Autodesk Inventor part; units mm, degrees
ref_plane "YZ Plane" through (0, 0, 0) normal (1, 0, 0) x (0, 1, 0)
ref_plane "XZ Plane" through (0, 0, 0) normal (0, 1, 0) x (-1, 0, 0)
ref_plane "XY Plane" through (0, 0, 0) normal (0, 0, 1) x (1, 0, 0)
sketch "Sketch1" plane through (0, 0, 0) normal (0, 1, 0) x (-1, 0, 0)
  line L0 (0, 0) -> (-358.4448, 0)
  line L1 (0, 0) -> (-358.4448, 0) construction
  line L2 (0, 0) -> (-358.4448, 0) construction
  line L3 (0, 25.4) -> (-358.4448, 25.4)
  line L4 (-358.4448, -25.4) -> (0, -25.4)
  arc A0 (0, -25.4) -> (0, 25.4) centre (0, 0) ccw
  arc A1 (-358.4448, 25.4) -> (-358.4448, -25.4) centre (-358.4448, 0) ccw
  circle A2 centre (0, 0) radius 14.2875
  circle A3 centre (-358.4448, 0) radius 14.2875
  point P0 (-179.2224, 0)
  point P1 (-179.2224, 0)
  dimension "d0" = 358.4448
  dimension "d8" = 50.8
  dimension "d9" = 28.575
  dimension "d10" = 28.575
extrude "Extrusion1" add sketch "Sketch1" along normal blind 6.35
properties part number "4-bar intake (14.112) bar"
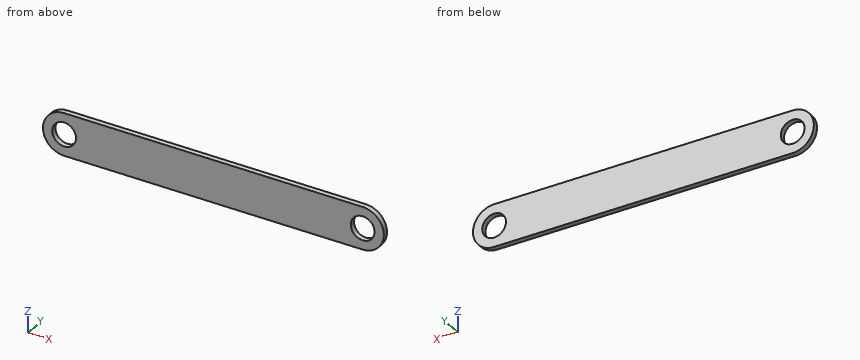
CAD build for the part. Positions are in the model's coordinates, mm. Give positions to 0.01 mm unless a question says otherwise; leave off trailing zeros. Write each loop counter-clockwise with the first axis right and the second up, starting at its lowest first coordinate (ties: lowest second). Pieces come first, ordered by that corner, then holes. Notation, with made-up numbers: M 11.5,46.5 L 64.5,46.5 A32 ccw 64.5,84.5 Z; hole C 18,39 d10. An arc over 180 degrees is marked long. Return JSON: item names as keys, results as strings. Group by question number.
(1) Drill centre lines: L1, parallel to X at y = 1.5, z = 1; L2, parallel to Z at x = 0, y = 2.5; L3, parallel to X at y = 5.75, z = -2. Where is each one in solid material? Low to high. Write a range as [from, to].
(2) Band-saw the part on A-A (z = 0). Give the cut face in (x, y).
(3) Flat gauge pins, fed straight in: pin 1 Ø23 at (x, z) = (0, 0) entering from +Y; pin 2 Ø2 at (y, z) = (2.5, -19) entering from -X; pin 3 Ø1.5 at (y, z) = (1, -19) entering from +X; pin 4 Ø1 at (y, z) = (4, 5.5) entering from +X. Where does each tip first touch, or does it go through?
(4) Band-saw the part on B-B (y = 1.5). Give the cut face in (x, z) (1 decimal), and give its area (3 significant figures).
(5) Band-saw the part on C-C (z = 18.5). Give the cut face in (x, y), and give its area (3 significant figures).
Entries:
{
 "1": {"L1": "x = [-25.38, -14.25], [14.25, 344.19], [372.7, 383.83]", "L2": "z = [-25.4, -14.29], [14.29, 25.4]", "L3": "x = [-25.32, -14.15], [14.15, 344.3], [372.59, 383.77]"},
 "2": {"outline": "M -25.4,0 L -14.29,0 L -14.29,6.35 L -25.4,6.35 Z; M 14.29,0 L 344.16,0 L 344.16,6.35 L 14.29,6.35 Z; M 372.73,0 L 383.84,0 L 383.84,6.35 L 372.73,6.35 Z"},
 "3": {"pin 1": "passes through", "pin 2": "stops at x = -17.92", "pin 3": "stops at x = 376.11", "pin 4": "stops at x = 383.35"},
 "4": {"outline": "M 0,-25.4 L 358.4,-25.4 A25.4 ccw 358.4,25.4 L 0,25.4 A25.4 ccw Z; hole C 0,0 d28.6; hole C 358.4,0 d28.6", "area": "19,000 mm^2"},
 "5": {"outline": "M -17.4,0 L 375.85,0 L 375.85,6.35 L -17.4,6.35 Z", "area": "2,500 mm^2"}
}
